from build123d import *

# Parameters (mm, degrees)
F0_R      = 25
F1_DEPTH  = 26
F3_DEPTH  = 20
F5_DEPTH  = 5.7
F7_DEPTH  = 5.9
F6_R      = 12.5
F8_DEPTH  = 26.001
F9_W      = 112
F9_H      = 56
F10_DEPTH = 17
F11_W     = 12
F11_H     = 28.827018
F12_DEPTH = 37.8
F14_DEPTH = 61.850929
F15_R     = 5
F16_DEPTH = 17.001
F18_DEPTH = 57.901
F19_R     = 4
F20_DEPTH = 25.001


with BuildPart() as f1:
    # F0 (on Front) → F1 (new body)
    with BuildSketch(Plane.XZ):
        Circle(F0_R)
    extrude(amount=F1_DEPTH)

    # F2 (on face) → F3 (join)
    with BuildSketch(Plane.XZ.offset(26)):
        Polygon((-25, 0), (-56, -74), (56, -74), (25, 0), align=None)
    extrude(amount=-F3_DEPTH)

    # F4 (on face) → F5 (cut)
    with BuildSketch(Plane.XZ.offset(26)):
        with BuildLine():
            ThreePointArc((25, 0), (0, -25.118919), (-25, 0))
            Line((-25, 0), (-56, -74))
            Line((-56, -74), (56, -74))
            Line((56, -74), (25, 0))
        make_face()
    extrude(amount=-F5_DEPTH, mode=Mode.SUBTRACT)

    # F4 (on face) → F7 (cut)
    with BuildSketch(Plane.XZ.offset(26)):
        with BuildLine():
            ThreePointArc((25, 0), (0, -25.118919), (-25, 0))
            Line((-25, 0), (-56, -74))
            Line((-56, -74), (56, -74))
            Line((56, -74), (25, 0))
        make_face()
    extrude(amount=-F7_DEPTH, mode=Mode.SUBTRACT)

    # F6 (on face) → F8 (cut, through all)
    with BuildSketch(Plane.XZ.offset(26)):
        Circle(F6_R)
    extrude(amount=-F8_DEPTH, mode=Mode.SUBTRACT)

    # F9 (on face) → F10 (join)
    with BuildSketch(Plane(origin=(0, 0, -74), x_dir=(1, 0, 0), z_dir=(0, 0, -1))):
        with Locations((0, -3.9)):
            Rectangle(F9_W, F9_H)
    extrude(amount=F10_DEPTH)

    # F11 (on face) → F12 (join)
    with BuildSketch(Plane(origin=(0, -6, 0), x_dir=(-1, 0, 0), z_dir=(0, 1, 0))):
        with Locations((-0.150071, -59.586491)):
            Rectangle(F11_W, F11_H)
    extrude(amount=F12_DEPTH)

    # F13 (on face) → F14 (cut, through all)
    with BuildSketch(Plane(origin=(-5.849929, 0, 0), x_dir=(0, -1, 0), z_dir=(-1, 0, 0))):
        Polygon((-31.8, -74), (6, -45.172982), (-31.8, -45.172982), align=None)
    extrude(amount=-F14_DEPTH, mode=Mode.SUBTRACT)

    # F15 (on face) → F16 (cut, through all)
    with BuildSketch(Plane.XY.offset(-74)):
        with Locations((-44, 13.9)):
            Circle(F15_R)
        with Locations((44, 13.9)):
            Circle(F15_R)
    extrude(amount=-F16_DEPTH, mode=Mode.SUBTRACT)

    # F17 (on face) → F18 (cut, through all)
    with BuildSketch(Plane(origin=(0, 31.9, 0), x_dir=(-1, 0, 0), z_dir=(0, 1, 0))):
        with BuildLine():
            Line((-31, -91), (31, -91))
            ThreePointArc((31, -91), (31.151032, -88.462802), (29.300669, -86.720292))
            Line((29.300669, -86.720292), (-29.08097, -86.498646))
            ThreePointArc((-29.08097, -86.498646), (-31.203205, -88.253629), (-31, -91))
        make_face()
    extrude(amount=-F18_DEPTH, mode=Mode.SUBTRACT)

    # F19 (on Top) → F20 (cut, through all)
    with BuildSketch(Plane.XY):
        with Locations((0, -13)):
            Circle(F19_R)
    extrude(amount=F20_DEPTH, mode=Mode.SUBTRACT)


solid = f1.part
Geometry check sheet. Reference: the model listing, model coordinates, mm. A direction names the side the tool comes from. Round coordinates to 2 decimals unless told otherwise and drop trailing zeros. Write each loop counter-clockwise with the first axis right and the second up, starting at its lowest first coordinate (ties: lowest second). Pieces come first, ordered by that corner, then holes. Notation, with made-up numbers: (65.25, -17) -> (96.25, -17) arc R16 ccw to (96.25, 6) -> close; hole circle Ø10 at (20.5, 45). An arc over 180 degrees is marked (long way). One line per item, written item: value. Start each with the question number.
(1) Cross-section at B-B, the plane z = 5. Record the cut outline in (x, y), and give its area (3 significant figures).
(2) Draft check along Z on faces 6 (the flat face through (-11.5, 0, 5.9)), 7 (the cylindrical face through (-3.255, -9.929, 24.787)), 8 (the flat face through (43, 4, -91)), 9 (the cylindrical face through (0.551, -23.091, -25.113)). Enter one of: +Z half, -Z half, draft (parallel to the pull), parting line (faces both ways), or undercut.
(3) Go/stop test with flat-tipped pins: pin 1 Ø4.5 at (x, y) = (4.5, -21.5) entering from +Z; pin 2 Ø5 at (x, y) = (0, -13) entering from -Z; pin 3 Ø4 at (x, y) = (-1.5, 23) entering from +Z. Record where each tip stops, or that it passes through.
(4) Cross-section at C-C, the plane x = 0. Record the cut outline in (y, z), and give its area (3 significant figures).
(5) Scan lines: line 1 (Y direction, x = 44, z = -86.5); line 2 (Z direction, x = 27, y = -3.5); line 3 (Y direction, x = -33, z = -22). Record each from-to range of solid material in increasing order. Write a range as [from, to].
(6) Cross-section at D-D, the plane x = -44. Record the cut outline in (y, z).
(7) Cross-section at A-A, the plane y = -4.5. Record the cut outline in (x, z), and give its area (3 significant figures).
(8) Access from +Z, -Z, +X, -X, +Y, -Y to the whole of each face (thin tool, end or side, straight path). Record for faces 1 (the cylindrical face through (31.19, 4.29, -88.22)), 2 (the flat face through (-1, -22, -74)), 3 (the flat face through (6.15, 8, -63)), 4 (the flat face through (-1, -6, -45)), 5 (the cylindrical face through (-48, 10.9, -82.4)).
Answer:
1. outline: (-24.49, -26) -> (-11.46, -26) -> (-11.46, 0) -> (-24.49, 0) -> close; (11.46, -26) -> (24.49, -26) -> (24.49, 0) -> (11.46, 0) -> close
1. area: 678 mm²
2. face 6: draft
2. face 7: undercut
2. face 8: -Z half
2. face 9: undercut
3. pin 1: z = 24.9
3. pin 2: z = -86.62
3. pin 3: z = -65.76
4. outline: (-26, -25.12) -> (-20.1, -25.12) -> (-20.1, -74) -> (-24.1, -74) -> (-24.1, -86.61) -> (31.9, -86.61) -> (31.9, -74) -> (31.8, -74) -> (-6, -45.17) -> (-6, -25) -> (0, -25) -> (0, -12.5) -> (-26, -12.5) -> close; (-26, 12.5) -> (-17, 12.5) -> (-17, 25) -> (-26, 25) -> close; (-9, 12.5) -> (0, 12.5) -> (0, 25) -> (-9, 25) -> close
4. area: 2,490 mm²
5. line 1: [-24.1, 8.9], [18.9, 31.9]
5. line 2: [-86.51, -74]
5. line 3: [-20.1, -6]
6. outline: (-24.1, -91) -> (8.9, -91) -> (8.9, -74) -> (-6, -74) -> (-6, -45.35) -> (-20.1, -45.35) -> (-20.1, -74) -> (-24.1, -74) -> close; (18.9, -91) -> (31.9, -91) -> (31.9, -74) -> (18.9, -74) -> close
7. outline: (-56, -91) -> (-31, -91) arc R3 cw to (-29.3, -86.72) -> (29.08, -86.5) arc R3 cw to (31, -91) -> (56, -91) -> (56, -74) -> (6.15, -74) -> (6.15, -46.32) -> (-5.85, -46.32) -> (-5.85, -74) -> (-56, -74) -> close; circle Ø50 at (0, 0); hole circle Ø25 at (0, 0)
7. area: 3,440 mm²
8. face 1: +Y, -Y
8. face 2: +X, -X, -Y
8. face 3: +X, +Y
8. face 4: +Y
8. face 5: +Z, -Z
